from build123d import *

# Parameters (mm, degrees)
SKETCH2_W           = 203.2
SKETCH2_H           = 101.6
BOSS_EXTRUDE1_DEPTH = 19.558
FILLET1_R           = 10
FILLET2_R           = 10
FILLET3_R           = 10
FILLET4_R           = 10
SKETCH3_R           = 4.445
BOSS_EXTRUDE3_DEPTH = 24.13
SKETCH4_R           = 19.05
CUT_EXTRUDE1_DEPTH  = 2.54


with BuildPart() as part:
    # Sketch2 → Boss-Extrude1 (new body)
    with BuildSketch(Plane(origin=(-97.482495003, 0, 34.735141898), x_dir=(1, 0, 0), z_dir=(0, 1, 0))):
        with Locations((-19.545959724, 34.347881976)):
            Rectangle(SKETCH2_W, SKETCH2_H)
    extrude(amount=BOSS_EXTRUDE1_DEPTH)

    # Fillet1
    fillet1_edges = [part.edges().sort_by_distance(p)[0] for p in [
        (-15.428454726, 9.779, 51.187259921),
    ]]
    fillet(fillet1_edges, radius=FILLET1_R)

    # Fillet2
    fillet2_edges = [part.edges().sort_by_distance(p)[0] for p in [
        (-218.628454726, 9.779, -50.412740079),
    ]]
    fillet(fillet2_edges, radius=FILLET2_R)

    # Fillet3
    fillet3_edges = [part.edges().sort_by_distance(p)[0] for p in [
        (-218.628454726, 9.779, 51.187259921),
    ]]
    fillet(fillet3_edges, radius=FILLET3_R)

    # Fillet4
    fillet4_edges = [part.edges().sort_by_distance(p)[0] for p in [
        (-15.428454726, 9.779, -50.412740079),
    ]]
    fillet(fillet4_edges, radius=FILLET4_R)

    # Sketch3 → Boss-Extrude3 (add)
    with BuildSketch(Plane(origin=(0, 0, -50.412740079), x_dir=(-1, 0, 0), z_dir=(0, 0, -1))):
        with Locations(Location((46.871325594, 9.049463129, 0), (0, 0, 180))):
            Circle(SKETCH3_R)
    boss_extrude3 = extrude(amount=BOSS_EXTRUDE3_DEPTH)

    # Mirror2: Boss-Extrude3 across plane
    add(boss_extrude3.mirror(Plane.XY))

    # Sketch4 → Cut-Extrude1 (cut)
    with BuildSketch(Plane.XZ):
        with Locations(Location((-175.512993917, 2.188610614, 0), (0, 0, 270))):
            Circle(SKETCH4_R)
    extrude(amount=-CUT_EXTRUDE1_DEPTH, mode=Mode.SUBTRACT)


solid = part.part
The listing builds one solid part. Answer for the finished solid, in the listing's coordinates (mm). A direction names the side the tool comes from. Coordinates: 2 decimals unless noted, no trailing zeros. Loops run counter-clockwise (first coordinate to the right, second up) from the corner with the lowest first, then second, coordinate; pieces in that order, holes last. Notation, with made-up numbers: M -34.5,4.5 L -12.5,4.5 A10 ccw -12.5,16.5 Z; hole C -27.5,21.5 d7. An arc over 180 degrees is marked long. Answer in a Markdown table with one row per item.
1) Find section C-C (y = 7). Determine the outline of the cut face in (x, z), then the cut area to 3 significant figures.
Answers below:
| item | result |
|---|---|
| outline | M -218.63,-40.41 A10 ccw -208.63,-50.41 L -50.82,-50.41 L -50.82,-74.54 L -42.93,-74.54 L -42.93,-50.41 L -25.43,-50.41 A10 ccw -15.43,-40.41 L -15.43,41.19 A10 ccw -25.43,51.19 L -42.93,51.19 L -42.93,74.54 L -50.82,74.54 L -50.82,51.19 L -208.63,51.19 A10 ccw -218.63,41.19 Z |
| area | 20,900 mm^2 |
2) Which of the six approach directions +Z, -Z, +X, -X, +Y, -Y give full straight-line access (tool end or side, diameter ignored) to faces 4 (the cylindrical face through (-51.31, 8.85, -62.31)), 5 (the cylindrical face through (-192.414, 1.252, -6.602)), 6 (the cylindrical face through (-51.31, 8.85, 62.7))?
Answers below:
| item | result |
|---|---|
| face 4 | -Z |
| face 5 | -Y |
| face 6 | +Z |
3) Find section D-D (x = -187). Determine the outline of the cut face in (y, z), then the cut area to 3 significant figures.
Answers below:
| item | result |
|---|---|
| outline | M 0,-50.41 L 19.56,-50.41 L 19.56,51.19 L 0,51.19 L 0,17.39 L 2.54,17.39 L 2.54,-13.01 L 0,-13.01 Z |
| area | 1,910 mm^2 |
4) Given pin 1 (5 mm diameter, centred on x = -184, z = 8, fed in from -Y); pin 2 (6 mm diameter, centred on x = -167, y = 17, fed in from -Z), each flat-ended and moving along its own axis, determine where each tip first touches the part or whether it passes through.
Answers below:
| item | result |
|---|---|
| pin 1 | y = 2.54 |
| pin 2 | z = -50.41 |
5) Find section B-B (z = -3). Determine the outline of the cut face in (x, y), then the cut area to 3 significant figures.
Answers below:
| item | result |
|---|---|
| outline | M -218.63,0 L -193.84,0 L -193.84,2.54 L -157.18,2.54 L -157.18,0 L -15.43,0 L -15.43,19.56 L -218.63,19.56 Z |
| area | 3,880 mm^2 |
6) Find the intervals of material crossed by probe 1 along X at (y, z) = (1.5, 1.5); probe 2 along Z at (x, y) = (-184, 8.75); probe 3 along X at (y, z) = (6.25, -53), in increasing order.
Answers below:
| item | result |
|---|---|
| probe 1 | -218.63 to -194.55, -156.48 to -15.43 |
| probe 2 | -50.41 to 51.19 |
| probe 3 | -50.32 to -43.42 |
7) Find section A-A (x = -84). Determine the outline of the cut face in (y, z).
Answers below:
| item | result |
|---|---|
| outline | M 0,-50.41 L 19.56,-50.41 L 19.56,51.19 L 0,51.19 Z |
8) Determine the mould class of faces 1 (the flat face through (-118, 0, 0)), 2 (the flat face through (-175, 2.54, 2)), 3 (the flat face through (-15.428, 10, 1)) for opening direction X: released by +X, released by -X, zero draft, split by the parting line, or undercut.
Answers below:
| item | result |
|---|---|
| face 1 | zero draft |
| face 2 | undercut |
| face 3 | released by +X |
